Check sheet for the modelled part. Datum: model origin and axes. Units: mm. A direction names the side the tool comes from. Round coordinates to 2 decimals unless told otherwise and drop trailing zeros. Loops run counter-clockwise (first coordinate to the right, second up) from the corner with the lowest first, then second, coordinate; pieces in that order, holes last. Notation, with made-up numbers: (-7.5, -13) - (28.5, -13) arc R25 ccw to (28.5, 13) - close; hole circle Ø9 at (16.25, -18.75). An arc over 180 degrees is marked (long way). Return JSON: item names as keys, results as strings.
from build123d import *

# Parameters (mm, degrees)
BOSS_EXTRUDE1_DEPTH = 10


with BuildPart() as part:
    # Sketch1 → Boss-Extrude1 (new body)
    with BuildSketch(Plane(origin=(0, 0, 0), x_dir=(1, 0, 0), z_dir=(0, 1, 0))):
        with BuildLine():
            Line((0, 0), (0, 20))
            ThreePointArc((0, 20), (2.5, 22.5), (5, 20))
            Line((5, 20), (5, 0))
            Line((5, 0), (10, 0))
            Line((10, 0), (10, 30))
            Line((10, 30), (35, 30))
            Line((35, 30), (35, 0))
            Line((35, 0), (40, 0))
            Line((40, 0), (40, 20))
            ThreePointArc((40, 20), (42.5, 22.5), (45, 20))
            Line((45, 20), (45, 0))
            Line((45, 0), (50, 0))
            Line((50, 0), (50, 30))
            Line((50, 30), (75, 30))
            Line((75, 30), (75, 0))
            Line((75, 0), (80, 0))
            Line((80, 0), (80, 20))
            ThreePointArc((80, 20), (82.5, 22.5), (85, 20))
            Line((85, 20), (85, 0))
            Line((85, 0), (90, 0))
            Line((90, 0), (90, 30))
            Line((90, 30), (115, 30))
            Line((115, 30), (115, 0))
            Line((115, 0), (120, 0))
            Line((120, 0), (120, 20))
            ThreePointArc((120, 20), (122.5, 22.5), (125, 20))
            Line((125, 20), (125, 0))
            Line((125, 0), (130, 0))
            Line((130, 0), (130, 30))
            Line((130, 30), (155, 30))
            Line((155, 30), (155, 0))
            Line((155, 0), (160, 0))
            Line((160, 0), (160, 20))
            ThreePointArc((160, 20), (162.5, 22.5), (165, 20))
            Line((165, 20), (165, 0))
            Line((165, 0), (170, 0))
            Line((170, 0), (170, 30))
            Line((170, 30), (195, 30))
            Line((195, 30), (195, 0))
            Line((195, 0), (200, 0))
            Line((200, 0), (200, 20))
            ThreePointArc((200, 20), (202.5, 22.5), (205, 20))
            Line((205, 20), (205, 0))
            Line((205, 0), (210, 0))
            Line((210, 0), (210, 30))
            Line((210, 30), (235, 30))
            Line((235, 30), (235, 0))
            Line((235, 0), (240, 0))
            Line((240, 0), (240, 20))
            ThreePointArc((240, 20), (242.5, 22.5), (245, 20))
            Line((245, 20), (245, 0))
            Line((245, 0), (250, 0))
            Line((250, 0), (250, 30))
            Line((250, 30), (250, 50))
            Line((250, 50), (-5, 50))
            Line((-5, 50), (-5, 30))
            Line((-5, 30), (-5, 0))
            Line((-5, 0), (0, 0))
        make_face()
    extrude(amount=BOSS_EXTRUDE1_DEPTH)


solid = part.part
Q1. Tool access check on faces 3 (the face through (124, 5, -50)), 4 (the face through (50, 5, -15)). Record the directions out of +Z, -Z, +X, -X, +Y, -Y that give a thin tool (end or side, any length) a straight path to the whole face; none if there is none.
Answer key:
{"face 3": "-Z, +X, -X, +Y, -Y", "face 4": "+Z, +Y, -Y"}
Q2. Scan lines: probe 1 along Z at (x, y) = (67.5, 9.75); probe 2 along Z at (x, y) = (83, 1.75). Record each from-to range of solid material in increasing order. Write a range as [from, to].
Answer key:
{"probe 1": "z = [-50, -30]", "probe 2": "z = [-50, -22.45]"}
Q3. Sectioned sample at A-A (z = -16.5). State how many separate pieces and enclosed holes the cut face has, plus the area to 3 significant figures.
Answer key:
{"separate pieces": "14", "enclosed holes": "0", "area": "700 mm²"}
Q4. Draft check along X on faces 1 (the face through (207, 5, 0)), 2 (the face through (200, 5, -10)). Enter one of: released by +X, released by -X, zero draft, split by the parting line, or undercut.
Answer key:
{"face 1": "zero draft", "face 2": "undercut"}
Q5. Depth check by flat-ended pin: P1, Ø5, axis at x = 61.5, y = 4, coming from the +Z side; P2, Ø1, axis at x = 211, z = -7, coming from the +Y side; P3, Ø4, axis at x = 129, y = 8, coming from the +Z side. Enter the tip coordinate at first touch or a pass-through.
Answer key:
{"P1": "stops at z = -30", "P2": "passes through", "P3": "stops at z = 0"}
Q6. Sectioned sample at B-B (x = 42.5). Enter the section's corners in (y, z).
Answer key:
{"outline": "(0, -50) - (10, -50) - (10, -22.5) - (0, -22.5) - close"}
